Design review of the part built by this model. Coordinates are the model's own, in mm. Face numbers are marked on the shaded views. A direction names the side the tool comes from. Coordinates: 2 decimals unless noted, no trailing zeros. Loops run counter-clockwise (first coordinate to the right, second up) from the corner with the lowest first, then second, coordinate; pieces in that order, holes last. Notation, with made-up numbers: (7, -22) - (58, -22) arc R12 ccw to (58, -13) - close; hole circle Ø3 at (74, -22.75). An arc over 180 degrees is marked (long way). Return JSON: item names as keys, results as strings. Group by question number.
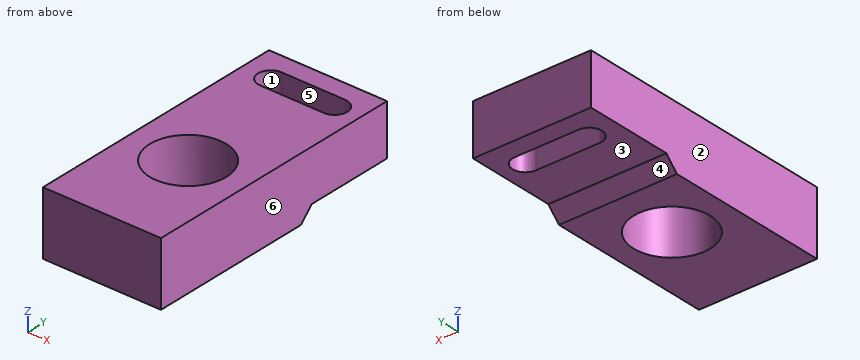
from build123d import *

# Parameters (mm, degrees)
SKETCH011_W     = 9.25
SKETCH011_H     = 21
SKETCH011_R     = 3
PAD006_DEPTH    = 5
SKETCH021_W     = 9.25
SKETCH021_H     = 7
POCKET006_DEPTH = 1
CHAMFER_SIZE    = 0.99


with BuildPart() as part:
    # Sketch011 → Pad006 (new body)
    with BuildSketch(Plane(origin=(16, -15, -11.5), x_dir=(1, 0, 0), z_dir=(0, 0, 1))):
        with Locations((0, 2.5)):
            Rectangle(SKETCH011_W, SKETCH011_H)
        Circle(SKETCH011_R, mode=Mode.SUBTRACT)
        with BuildLine():
            ThreePointArc((-2.375, 11.5), (-3.375, 10.5), (-2.375, 9.5))
            Line((-2.375, 9.5), (2.625, 9.5))
            ThreePointArc((2.625, 9.5), (3.625, 10.5), (2.625, 11.5))
            Line((-2.375, 11.5), (2.625, 11.5))
        make_face(mode=Mode.SUBTRACT)
    extrude(amount=-PAD006_DEPTH)

    # Sketch021 → Pocket006 (cut)
    with BuildSketch(Plane(origin=(16, -15, -16.5), x_dir=(1, 0, 0), z_dir=(0, 0, -1))):
        with Locations((0, -9.5)):
            Rectangle(SKETCH021_W, SKETCH021_H)
    extrude(amount=-POCKET006_DEPTH, mode=Mode.SUBTRACT)

    # Chamfer
    chamfer_edges = [part.edges().sort_by_distance(p)[0] for p in [
        (16, -9, -16.5),
    ]]
    chamfer(chamfer_edges, length=CHAMFER_SIZE)


solid = part.part
Item 1: Add section C-C (z = -14.6). State the section outline as (x, y) points (3 decimals), then the cut area to 3 significant figures.
Item 2: Add section A-A (y = -15). State the section outline as (x, z) points (3 decimals).
Item 3: For the marked faces 1, 2 and 3, list the 3-axis set-ups (+Z, -Z, +X, -X, +Y, -Y) from which the entire face can be reached by the end or side of a thin tool; tool diameter is ignored.
Item 4: To check wall thickness, follow line 1 (Y direction, x = 16, z = -13.75); line 2 (Y direction, x = 16.75, z = -11.95); line 3 (Y direction, x = 19.25, z = -13.2). State the ranges of each line that lie inside material, in increasing order. Write a range as from..to.
Item 5: Add section D-D (y = -4.5). State the section outline as (x, z) points (3 decimals).
Item 6: Draft analysis for pull direction Y (two halves, no side actions). For the marked faces 4, 5 and 6, state which applies: pulls with the +Y half, pulls with the -Y half, needs draft (parallel to the pull), parting line crosses it, or undercut.
Item 7: For P1, Ø1, axis at x = 14, y = -7, coming from the -Z side, flat-tipped, find the tip position at first contact; note if it passes through.
Item 8: Add section B-B (x = 16). Give the number of separate pieces and of enclosed holes in the cut face, then the cut area to 3 significant figures.
Answers below:
{
 "1": {"outline": "(11.375, -23) - (20.625, -23) - (20.625, -2) - (11.375, -2) - close; hole circle Ø6 at (16, -15); hole (13.625, -5.5) - (18.625, -5.5) arc R1 ccw to (18.625, -3.5) - (13.625, -3.5) arc R1 ccw to start", "area": "153 mm^2"},
 "2": {"outline": "(11.375, -16.5) - (13, -16.5) - (13, -11.5) - (11.375, -11.5) - close; (19, -16.5) - (20.625, -16.5) - (20.625, -11.5) - (19, -11.5) - close"},
 "3": {"face 1": "+Z, -Z", "face 2": "+Z, -Z, -X, +Y, -Y", "face 3": "-Z, +X, -X, +Y"},
 "4": {"line 1": "y = -23..-18, -12..-5.5, -3.5..-2", "line 2": "y = -23..-17.9, -12.1..-5.5, -3.5..-2", "line 3": "y = -23..-5.28, -3.72..-2"},
 "5": {"outline": "(11.375, -15.5) - (12.625, -15.5) - (12.625, -11.5) - (11.375, -11.5) - close; (19.625, -15.5) - (20.625, -15.5) - (20.625, -11.5) - (19.625, -11.5) - close"},
 "6": {"face 4": "pulls with the +Y half", "face 5": "undercut", "face 6": "needs draft"},
 "7": {"P1": "stops at z = -15.5"},
 "8": {"separate pieces": "3", "enclosed holes": "0", "area": "59.5 mm^2"}
}
